from build123d import *

# Parameters (mm, degrees)
SKETCH_1_W              = 16
SKETCH_1_H              = 3
EXTRUDE_1_DEPTH         = 10
SKETCH_2_W              = 30
SKETCH_2_H              = 20
EXTRUDE_2_DEPTH         = 3
HOLE_WIZARD_2_2_2_2_1_D = 2.2
FILLET_1_R              = 0.7
HOLE_WIZARD_2_2_2_2_2_D = 2.2


with BuildPart() as part:
    # 草图1 → 凸台-拉伸1 (new body)
    with BuildSketch(Plane.XY):
        with Locations((0, 1.5)):
            Rectangle(SKETCH_1_W, SKETCH_1_H)
    extrude(amount=-EXTRUDE_1_DEPTH)

    # 草图2 → 凸台-拉伸2 (add)
    with BuildSketch(Plane.XY):
        with Locations((7, 10)):
            Rectangle(SKETCH_2_W, SKETCH_2_H)
    extrude(amount=EXTRUDE_2_DEPTH)

    # Ø2.2 (2.2) 直径孔1 (through all)
    with Locations(Plane(origin=(0, 3, 0), x_dir=(1, 0, 0), z_dir=(0, 1, 0))):
        with Locations((-5, 5), (5, 5)):
            Hole(HOLE_WIZARD_2_2_2_2_1_D / 2)

    # 圆角1
    fillet_1_edges = [part.edges().sort_by_distance(p)[0] for p in [
        (8, 1.5, -10),
        (-8, 11.5, 0),
        (15, 0, 0),
        (22, 10, 0),
        (22, 0, 1.5),
        (7, 20, 0),
        (22, 20, 1.5),
        (-8, 10, 3),
        (7, 0, 3),
        (0, 3, -10),
        (22, 10, 3),
        (7, 20, 3),
        (-8, 1.5, -10),
        (0, 3, 0),
        (8, 1.5, 0),
        (-8, 3, -5),
        (8, 3, -5),
        (8, 0, -5),
        (-8, 0, -3.5),
        (0, 0, -10),
    ]]
    fillet(fillet_1_edges, radius=FILLET_1_R)

    # Ø2.2 (2.2) 直径孔2 (through all)
    with Locations(Plane(origin=(0, 0, 0), x_dir=(-1, 0, 0), z_dir=(0, 0, -1))):
        with Locations((-17, 12.52), (-7, 12.52), (3, 12.52)):
            Hole(HOLE_WIZARD_2_2_2_2_2_D / 2)


solid = part.part
Geometry: final body of the model. Coordinates: model frame, mm. A direction names the side the tool comes from. Give positions to 0.01 mm unless a question says otherwise; leave off trailing zeros. Order: outer loops, then holes, each group sorted by start corner. A loop starts at its lowest first (then second) coordinate and runs counter-clockwise, first axis right, second up. Notation, with made-up numbers: (48.5, 58.5) -> (71.5, 58.5) arc R13 ccw to (71.5, 62.5) -> close; hole circle Ø5 at (-39.5, 69). An arc over 180 degrees is marked (long way). Write each question's results on one line, items separated by ' | '.
1) Cut plane A-A (z = -5). Output: boundary loops of the cut face in (x, y).
Geometry says:
outline: (-8, 0.7) arc R0.7 ccw to (-7.3, 0) -> (-6.1, 0) -> (-6.1, 3) -> (-7.3, 3) arc R0.7 ccw to (-8, 2.3) -> close; (-3.9, 0) -> (3.9, 0) -> (3.9, 3) -> (-3.9, 3) -> close; (6.1, 0) -> (7.3, 0) arc R0.7 ccw to (8, 0.7) -> (8, 2.3) arc R0.7 ccw to (7.3, 3) -> (6.1, 3) -> close
2) Set-up query: faces 1 (the face through (8, 1, -5)), 2 (the face through (0, 0, -4)). Return all of +Z, -Z, +X, -X, +Y, -Y with unobstructed straight access to the full face (end or side cutting, diameter ignored); none if empty.
Geometry says:
face 1: -Z, +X, +Y, -Y | face 2: +Z, -Z, +X, -X, -Y
3) First-contact query: pin 1 Ø3 at (x, y) = (7, 12.52) entering from -Z; pin 2 Ø3 at (x, z) = (5, -5) entering from +Y; pin 3 Ø1.8 at (y, z) = (1.5, -4) entering from +X; pin 4 Ø5 at (x, z) = (-0.5, 0) entering from +Y. Flat tips, straight axial feed; report the tip coordinate or a pass-through.
Geometry says:
pin 1: stops at z = 0 | pin 2: stops at y = 3 | pin 3: stops at x = 8 | pin 4: stops at y = 20
4) Cut plane D-D (z = -6.5). Output: boundary loops of the cut face in (x, y).
Geometry says:
outline: (-8, 0.7) arc R0.7 ccw to (-7.3, 0) -> (7.3, 0) arc R0.7 ccw to (8, 0.7) -> (8, 2.3) arc R0.7 ccw to (7.3, 3) -> (-7.3, 3) arc R0.7 ccw to (-8, 2.3) -> close
5) Draft query along Y for faces 3 (the face through (7.59, 13.45, 1.52)), 4 (the face through (0, 3, -5)), 5 (the face through (-4.189, 1.479, -5.743)). Return one class per face: released by +Y, released by -Y, zero draft, split by the parting line, or undercut.
Geometry says:
face 3: undercut | face 4: released by +Y | face 5: zero draft
6) Cut plane C-C (x = -5). Output: boundary loops of the cut face in (y, z).
Geometry says:
outline: (0, -9.3) arc R0.7 ccw to (0.7, -10) -> (2.3, -10) arc R0.7 ccw to (3, -9.3) -> (3, -6.1) -> (0, -6.1) -> close; (0, -3.9) -> (3, -3.9) -> (3, -0.7) arc R0.7 cw to (3.7, 0) -> (19.3, 0) arc R0.7 ccw to (20, 0.7) -> (20, 2.3) arc R0.7 ccw to (19.3, 3) -> (0.7, 3) arc R0.7 ccw to (0, 2.3) -> close
7) Cut plane B-B (y = 12.52). Output: boundary loops of the cut face in (x, z), and give its area (3 significant figures).
Geometry says:
outline: (-8, 0.7) arc R0.7 ccw to (-7.3, 0) -> (-4.1, 0) -> (-4.1, 3) -> (-7.3, 3) arc R0.7 ccw to (-8, 2.3) -> close; (-1.9, 0) -> (5.9, 0) -> (5.9, 3) -> (-1.9, 3) -> close; (8.1, 0) -> (15.9, 0) -> (15.9, 3) -> (8.1, 3) -> close; (18.1, 0) -> (21.3, 0) arc R0.7 ccw to (22, 0.7) -> (22, 2.3) arc R0.7 ccw to (21.3, 3) -> (18.1, 3) -> close | area: 69.8 mm²
8) Line query: line 1 along X through (y, z) = (0.9, -5); line 2 along Y through (x, z) = (-3, 1.55); line 3 along Y through (x, z) = (4, -3). Output: solid intervals per line, ascending.
Geometry says:
line 1: x = -8 to -6.1, -3.9 to 3.9, 6.1 to 8 | line 2: y = 0 to 11.42, 13.62 to 20 | line 3: y = 0 to 3
